```python
from build123d import *

# Parameters (mm, degrees)
F0_W     = 1185
F0_H     = 70
F1_DEPTH = 10
F2_W     = 86
F2_H     = 32
F3_DEPTH = 691
F4_W     = 32
F4_H     = 81
F5_DEPTH = 994
F6_W     = 70
F6_H     = 32
F6_W_2   = 230
F7_DEPTH = 294


with BuildPart() as f1:
    # F0 (on Top) → F1 (new body)
    with BuildSketch(Plane.XY):
        with Locations((592.5, 35)):
            Rectangle(F0_W, F0_H)
    extrude(amount=-F1_DEPTH)

    # F2 (on face) → F3 (join)
    with BuildSketch(Plane(origin=(0, 0, -10), x_dir=(1, 0, 0), z_dir=(0, 0, -1))):
        with Locations((52.5, -35)):
            Rectangle(F2_W, F2_H)
        with Locations((1132.5, -35)):
            Rectangle(F2_W, F2_H)
    extrude(amount=F3_DEPTH)

    # F4 (on face) → F5 (join, through all)
    with BuildSketch(Plane(origin=(1089.5, 0, 0), x_dir=(0, -1, 0), z_dir=(-1, 0, 0))):
        with Locations((-35, -50.5)):
            Rectangle(F4_W, F4_H)
        with Locations((-35, -425.5)):
            Rectangle(F4_W, F4_H)
    extrude(amount=F5_DEPTH)

    # F6 (on face) → F7 (join, through all)
    with BuildSketch(Plane.XY.offset(-385)):
        with Locations((958.5, 35)):
            Rectangle(F6_W, F6_H)
        with Locations((838.5, 35)):
            Rectangle(F6_W, F6_H)
        with Locations((592.5, 35)):
            Rectangle(F6_W_2, F6_H)
        with Locations((346.5, 35)):
            Rectangle(F6_W, F6_H)
        with Locations((226.5, 35)):
            Rectangle(F6_W, F6_H)
    extrude(amount=F7_DEPTH)


solid = f1.part
```
The model under review builds one solid part; all positions refer to its coordinate system, in mm. A direction names the side the tool comes from. Round coordinates to 2 decimals unless told otherwise and drop trailing zeros. Order: outer loops, then holes, each group sorted by start corner. A loop starts at its lowest first (then second) coordinate and runs counter-clockwise, first axis right, second up.
Item 1: To check wall thickness, follow probe 1 along X at (y, z) = (41.5, -555); probe 2 along X at (y, z) = (42, -433.5); probe 3 along Y at (x, z) = (725.5, -458). State the ranges of each line that lie inside material, in increasing order.
Working result:
probe 1: x = 9.5 to 95.5, 1089.5 to 1175.5
probe 2: x = 9.5 to 1175.5
probe 3: y = 19 to 51
Item 2: Draft analysis for pull direction X (two halves, no side actions). For faces 4 (the flat face through (287, 35, -91)), 5 (the flat face through (1175.5, 35, -351)), 6 (the flat face through (1132, 35, -701)), state which applies: released by +X, released by -X, zero draft, split by the parting line, or undercut.
Working result:
face 4: undercut
face 5: released by +X
face 6: zero draft
Item 3: Add section C-C, the plane z = -483. State the section outline as (x, y) points.
Working result:
outline: (9.5, 19) - (95.5, 19) - (95.5, 51) - (9.5, 51) - close; (1089.5, 19) - (1175.5, 19) - (1175.5, 51) - (1089.5, 51) - close
Item 4: Machinability: for faces 1 (the flat face through (1089.5, 35, -582)), 2 (the flat face through (707.5, 35, -240)), 3 (the flat face through (601, 51, -284)), which of the approach directions +Z, -Z, +X, -X, +Y, -Y give a long, thin tool a straight path to every point of the face, cutting with its end or side? Answer none if there is none.
Working result:
face 1: -Z, +Y, -Y
face 2: +Y, -Y
face 3: -Z, +X, -X, +Y
Item 5: For pin 1 (9.5 mm diameter, centred on y = 39.5, z = -584, fed in from +X); pin 2 (16 mm diameter, centred on x = 898, y = 35.5, fed in from -Z); pin 3 (16 mm diameter, centred on x = 1018.5, y = 40, fed in from +Z); pin 4 (16 mm diameter, centred on y = 40.5, z = -168.5, fed in from -X), all flat-tipped, find the tip position at first contact; note any pin that passes through.
Working result:
pin 1: stops at x = 1175.5
pin 2: stops at z = -466
pin 3: stops at z = 0
pin 4: stops at x = 9.5
Item 6: Add section B-B, the plane z = -365. State the section outline as (x, y) points.
Working result:
outline: (9.5, 19) - (95.5, 19) - (95.5, 51) - (9.5, 51) - close; (191.5, 19) - (261.5, 19) - (261.5, 51) - (191.5, 51) - close; (311.5, 19) - (381.5, 19) - (381.5, 51) - (311.5, 51) - close; (477.5, 19) - (707.5, 19) - (707.5, 51) - (477.5, 51) - close; (803.5, 19) - (873.5, 19) - (873.5, 51) - (803.5, 51) - close; (923.5, 19) - (993.5, 19) - (993.5, 51) - (923.5, 51) - close; (1089.5, 19) - (1175.5, 19) - (1175.5, 51) - (1089.5, 51) - close
Item 7: Add section A-A, the plane x = 776. State the section outline as (y, z) points, and give its area (3 significant figures).
Working result:
outline: (0, -10) - (19, -10) - (19, -91) - (51, -91) - (51, -10) - (70, -10) - (70, 0) - (0, 0) - close; (19, -466) - (51, -466) - (51, -385) - (19, -385) - close
area: 5,880 mm2
Item 8: Add section D-D, the plane x = 574.5. State the section outline as (y, z) points.
Working result:
outline: (0, -10) - (19, -10) - (19, -466) - (51, -466) - (51, -10) - (70, -10) - (70, 0) - (0, 0) - close
